Geometry check sheet. Reference: the model listing, model coordinates, mm. A direction names the side the tool comes from. Give positions to 0.01 mm unless a question says otherwise; leave off trailing zeros. Order: outer loops, then holes, each group sorted by start corner. A loop starts at its lowest first (then second) coordinate and runs counter-clockwise, first axis right, second up. Notation, with made-up numbers: M -33.75,-11.5 L 23.25,-11.5 A16 ccw 23.25,19.5 Z; hole C 29,41 d4. An arc over 180 degrees is marked long. Answer as CSV lines item,"result". Start each with the question number.
```python
from build123d import *

# Parameters (mm, degrees)
F0_W      = 93.7260054052
F0_H      = 73.1520000845
F1_DEPTH  = 10.16
F3_DEPTH  = 10.16
F5_DEPTH  = 10.16
F6_DEPTH  = 25.4
F7_W      = 10.1599991322
F7_H      = 1.7780002672
F8_DEPTH  = 2.286
F9_W      = 26.4160018414
F9_H      = 73.1520000845
F10_DEPTH = 127
F12_R     = 2.3962316347
F12_R_2   = 2.1849898249
F13_DEPTH = 2.54


with BuildPart() as f1:
    # F0 (on Front) → F1 (new body)
    with BuildSketch(Plane.XZ):
        with Locations((0.8890014142, -5.3366450593)):
            Rectangle(F0_W, F0_H)
    extrude(amount=F1_DEPTH)

    # F2 (on face) → F3 (cut)
    with BuildSketch(Plane.XZ.offset(10.16)):
        Polygon((47.7520041168, 31.239354983), (11.1760003492, 31.239354983), (47.7520041168, 21.5873550624), align=None)
    extrude(amount=-F3_DEPTH, mode=Mode.SUBTRACT)

    # F4 (on face) → F5 (cut)
    with BuildSketch(Plane.XZ.offset(10.16)):
        Polygon((8.6359996349, 24.1273548454), (-36.5759991109, 24.1273548454), (-35.813998431, 6.0933548957), (26.9239991903, 6.0933548957), align=None)
    extrude(amount=-F5_DEPTH, mode=Mode.SUBTRACT)

    # F6 (add): a face of the model
    f6_faces = [f1.faces().sort_by_distance(p)[0] for p in [
        (1.4948059303, -10.16, -9.7731364868),
    ]]
    extrude(f6_faces, amount=F6_DEPTH)

    # F7 (on face) → F8 (join)
    with BuildSketch(Plane.XZ.offset(35.56)):
        with Locations((-38.1000004709, -4.1936453199)):
            Rectangle(F7_W, F7_H)
    extrude(amount=F8_DEPTH)

    # F9 (on face) → F10 (cut)
    with BuildSketch(Plane(origin=(-45.9740012884, 0, 0), x_dir=(0, -1, 0), z_dir=(-1, 0, 0))):
        with Locations((13.2080009207, -5.3366450593)):
            Rectangle(F9_W, F9_H)
    extrude(amount=-F10_DEPTH, mode=Mode.SUBTRACT)

    # F12 (on face) → F13 (join)
    with BuildSketch(Plane(origin=(0, 0, -41.9126451015), x_dir=(1, 0, 0), z_dir=(0, 0, -1))):
        with Locations((43.8149981201, 31.4933545887)):
            Circle(F12_R)
        with Locations((43.8149981201, 31.4933545887)):
            Circle(F12_R_2, mode=Mode.SUBTRACT)
    extrude(amount=F13_DEPTH)


solid = f1.part
```
Item 1: Section check B-B on x = 7. Record the boundary of the cut face in (y, z).
Item 2: Section check A-A on y = -28. Record the boundary of the cut face in (x, z).
Item 3: Section check C-C on z = 14. Record the boundary of the cut face in (x, y).
Item 4: Depth check by flat-ended pin: pin 1 Ø1.4 at (y, z) = (-37, -4) entering from +X; pin 2 Ø2 at (x, z) = (15.5, -13) entering from -Y; pin 3 Ø4.5 at (x, y) = (22.5, -32.5) entering from -Z. Enter the tip coordinate at first touch or a pass-through.
Item 5: Scan lines: line 1 along Z through (x, y) = (-26, -29); line 2 along X through (y, z) = (-29.75, 8); line 3 along Y through (x, z) = (13, -5.5). Record each from-to range of solid material in increasing order.
Item 6: Draft check along X on faces 1 (the face through (-45.974, -31, -6)), 2 (the face through (0, -35.56, -13)), 3 (the face through (42.205, -32.97, -43.165)), 4 (the face through (-14, -31, 24.127)). Enter one of: pulls with the +X half, pulls with the -X half, needs draft (parallel to the pull), parting line crosses it, or undercut.
Item 7: Section check D-D on z = -36. Record the boundary of the cut face in (x, y), then the cut area to 3 significant figures.
Item 8: Access from +Z, -Z, +X, -X, +Y, -Y to the whole of each face (thin tool, end or side, straight path). Record for faces 5 (the face through (-38, -37, -3.305)), 6 (the face through (44, -31, -41.913)), 7 (the face through (-5, -31, 6.093)).
Numbers:
1,outline,"M -35.56,-41.91 L -26.42,-41.91 L -26.42,6.09 L -35.56,6.09 Z; M -35.56,24.13 L -26.42,24.13 L -26.42,31.24 L -35.56,31.24 Z"
2,outline,"M -45.97,-41.91 L 47.75,-41.91 L 47.75,21.59 L 11.18,31.24 L -45.97,31.24 Z; hole M -36.58,24.13 L -35.81,6.09 L 26.92,6.09 L 8.64,24.13 Z"
3,outline,"M -45.97,-35.56 L -36.15,-35.56 L -36.15,-26.42 L -45.97,-26.42 Z; M 18.91,-35.56 L 47.75,-35.56 L 47.75,-26.42 L 18.91,-26.42 Z"
4,pin 1,"x = -33.02"
4,pin 2,"y = -35.56"
4,pin 3,"z = -41.91"
5,line 1,"-41.91 to 6.09, 24.13 to 31.24"
5,line 2,"-45.97 to -35.89, 24.99 to 47.75"
5,line 3,"-35.56 to -26.42"
6,face 1,"pulls with the -X half"
6,face 2,"needs draft"
6,face 3,"undercut"
6,face 4,"undercut"
7,outline,"M -45.97,-35.56 L 47.75,-35.56 L 47.75,-26.42 L -45.97,-26.42 Z"
7,area,"857 mm2"
8,face 5,"+Z, +X, -X, -Y"
8,face 6,"-Z"
8,face 7,"+Y, -Y"
